from build123d import *

# Parameters (mm, degrees)
BOSS_EXTRUDE1_DEPTH      = 914.4
BOSS_EXTRUDE1_DEPTH_BACK = 914.4
SKETCH1_W                = 31.75
SKETCH1_H                = 31.75
SKETCH1_W_2              = 25.4
SKETCH1_H_2              = 25.4
FILLET1_R                = 1.5875
SKETCH5_W                = 25.4
SKETCH5_H                = 25.4
CUT_EXTRUDE1_DEPTH       = 1670.05


with BuildPart() as part:
    # Sketch1 → Boss-Extrude1 (new, two sides: drawn at the far end of the back side and taken through both)
    with BuildSketch(Plane.XY.offset(-BOSS_EXTRUDE1_DEPTH_BACK)):
        Rectangle(SKETCH1_W, SKETCH1_H)
        Rectangle(SKETCH1_W_2, SKETCH1_H_2, mode=Mode.SUBTRACT)
    extrude(amount=BOSS_EXTRUDE1_DEPTH + BOSS_EXTRUDE1_DEPTH_BACK)

    # Fillet1
    fillet1_edges = [part.edges().sort_by_distance(p)[0] for p in [
        (15.875, -15.875, 0),
        (-15.875, -15.875, 0),
        (-15.875, 15.875, 0),
        (15.875, 15.875, 0),
    ]]
    fillet(fillet1_edges, radius=FILLET1_R)

    # Sketch5 → Cut-Extrude1 (cut)
    with BuildSketch(Plane.XY.offset(914.4)):
        with BuildLine():
            Line((-14.2875, 15.875), (14.2875, 15.875))
            ThreePointArc((14.2875, 15.875), (15.410032015, 15.410032015), (15.875, 14.2875))
            Line((15.875, 14.2875), (15.875, -14.2875))
            ThreePointArc((15.875, -14.2875), (15.410032015, -15.410032015), (14.2875, -15.875))
            Line((14.2875, -15.875), (-14.2875, -15.875))
            ThreePointArc((-14.2875, -15.875), (-15.410032015, -15.410032015), (-15.875, -14.2875))
            Line((-15.875, -14.2875), (-15.875, 14.2875))
            ThreePointArc((-15.875, 14.2875), (-15.410032015, 15.410032015), (-14.2875, 15.875))
        make_face()
        Rectangle(SKETCH5_W, SKETCH5_H, mode=Mode.SUBTRACT)
    extrude(amount=-CUT_EXTRUDE1_DEPTH, mode=Mode.SUBTRACT)


solid = part.part
The listing builds one solid part. Answer for the finished solid, in the listing's coordinates (mm). A direction names the side the tool comes from. Round coordinates to 2 decimals unless told otherwise and drop trailing zeros. Order: outer loops, then holes, each group sorted by start corner. A loop starts at its lowest first (then second) coordinate and runs counter-clockwise, first axis right, second up. Notation, with made-up numbers: M 18.25,68.5 L 65.25,68.5 A30 cw 65.25,102.5 Z; hole C 88.25,6 d4. An arc over 180 degrees is marked long. Answer in a Markdown table with one row per item. Add a question column.
1) Which of the six approach directions +Z, -Z, +X, -X, +Y, -Y give full straight-line access (tool end or side, diameter ignored) to faces 4 (the face through (15.875, 0, -836)), 5 (the face through (12.7, 0, -836))?
2) Determine the mould class of faces 1 (the face through (0, -15.875, -836)), 2 (the face through (0, -12.7, -836)), 3 (the face through (14, 0, -755.65)) for opening direction Y: pulls with the +Y half, pulls with the -Y half, needs draft (parallel to the pull), parting line crosses it, or undercut.
3) The part is cut by section B-B on z = -821. Determine the outline of the cut face in (x, y) (1 decimal).
4) Consider line 1 along Y through (x, z) = (2.5, -784.5) (3 decimals). Determine where the line is inside the solid, lowest interval first. Write a range as from..to.
5) The part is cut by section A-A on x = 0. Determine the outline of the cut face in (y, z) (3 decimals).
Findings below:
| question | item | result |
|---|---|---|
| 1 | face 4 | +Z, -Z, +X, +Y, -Y |
| 1 | face 5 | +Z, -Z |
| 2 | face 1 | pulls with the -Y half |
| 2 | face 2 | undercut |
| 2 | face 3 | needs draft |
| 3 | outline | M -15.9,-14.3 A1.6 ccw -14.3,-15.9 L 14.3,-15.9 A1.6 ccw 15.9,-14.3 L 15.9,14.3 A1.6 ccw 14.3,15.9 L -14.3,15.9 A1.6 ccw -15.9,14.3 Z; hole M -12.7,-12.7 L 12.7,-12.7 L 12.7,12.7 L -12.7,12.7 Z |
| 4 | line 1 | y = -15.875..-12.7, 12.7..15.875 |
| 5 | outline | M -15.875,-914.4 L -12.7,-914.4 L -12.7,-755.65 L -15.875,-755.65 Z; M 12.7,-914.4 L 15.875,-914.4 L 15.875,-755.65 L 12.7,-755.65 Z |
